Design review of the part built by this model. Coordinates are the model's own, in mm. Face numbers are marked on the shaded views. A direction names the side the tool comes from. Coordinates: 2 decimals unless noted, no trailing zeros. Write each loop counter-clockwise with the first axis right and the second up, starting at its lowest first coordinate (ties: lowest second). Pieces come first, ordered by that corner, then holes.
Q1. Machinability: for the marked faces 1 and 2, which of the approach directions +Z, -Z, +X, -X, +Y, -Y give a long, thin tool a straight path to every point of the face, cutting with its end or side? Answer none if there is none.
Q2. Take a section at B-B (z = 0). Give the boundary of the cut face in (x, y).
Q3. Take a section at A-A (x = -6). Give the boundary of the cut face in (y, z), and give its area (3 significant figures).
Q4. Take a section at C-C (y = -0.5). Give the boundary of the cut face in (x, z).
Q5. For probe 1 along Y at (x, z) = (9, -6.25); probe 2 along X at (y, z) = (-22, -5); probe 3 along X at (y, z) = (-20.25, 2.5), list the stretches that pass through material, from the lowest coordinate up.
Q6. Insertion check: pin 1 (1.5 mm diameter, centred on x = -6.5, y = -20, fed in from +Z); pin 2 (6 mm diameter, centred on x = 11, y = -4.5, fed in from -Z); pin 3 (5 mm diameter, centred on y = -12, z = 4.5, fed in from -X). Each pin has a flat end and moves straight along its axis. Give the tip position at first contact, or say it passes through.
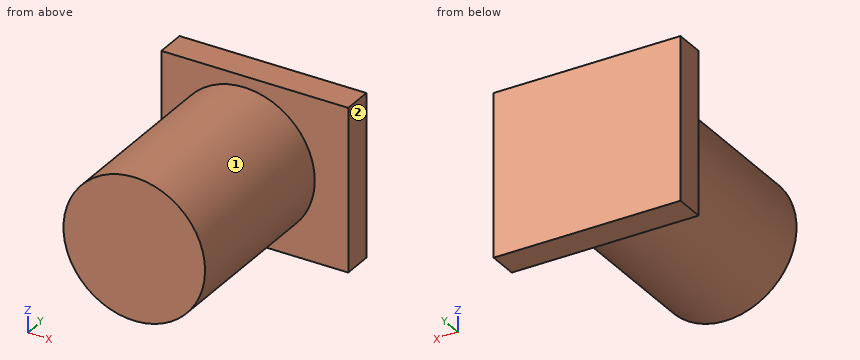
```python
from build123d import *

# Parameters (mm, degrees)
F0_R     = 10
F1_DEPTH = 25.4
F2_W     = 26.393833
F2_H     = 22.931724
F3_DEPTH = 4.2


with BuildPart() as f1:
    # F0 (on Front) → F1 (new body)
    with BuildSketch(Plane.XZ):
        Circle(F0_R)
    extrude(amount=F1_DEPTH)

    # F2 (on Front) → F3 (join)
    with BuildSketch(Plane.XZ):
        with Locations((1.531839, 0.090714)):
            Rectangle(F2_W, F2_H)
    extrude(amount=-F3_DEPTH)


solid = f1.part
```
Response:
1. face 1: -Y
1. face 2: +Z, -Z, +X, +Y, -Y
2. outline: (-11.67, 0) - (-10, 0) - (-10, -25.4) - (10, -25.4) - (10, 0) - (14.73, 0) - (14.73, 4.2) - (-11.67, 4.2) - close
3. outline: (-25.4, -8) - (0, -8) - (0, -11.38) - (4.2, -11.38) - (4.2, 11.56) - (0, 11.56) - (0, 8) - (-25.4, 8) - close
3. area: 503 mm2
4. outline: circle Ø20 at (0, 0)
5. probe 1: y = 0 to 4.2
5. probe 2: x = -8.66 to 8.66
5. probe 3: x = -9.68 to 9.68
6. pin 1: stops at z = 8.18
6. pin 2: stops at z = -6
6. pin 3: stops at x = -9.8
